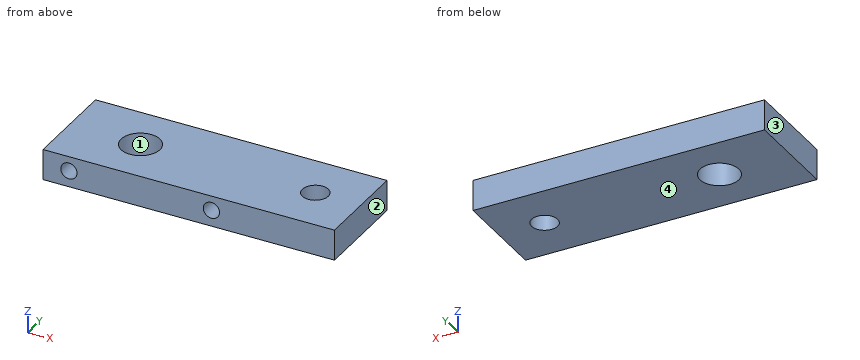
```python
from build123d import *

# Parameters (mm, degrees)
SKETCH1_W           = 90
SKETCH1_H           = 30
SKETCH1_R           = 6
SKETCH1_R_2         = 4
BOSS_EXTRUDE1_DEPTH = 9.5
SKETCH2_R           = 2.5
CUT_EXTRUDE1_DEPTH  = 15


with BuildPart() as part:
    # Sketch1 → Boss-Extrude1 (new body)
    with BuildSketch(Plane.XY):
        Rectangle(SKETCH1_W, SKETCH1_H)
        with Locations((-23, 0)):
            Circle(SKETCH1_R, mode=Mode.SUBTRACT)
        with Locations((30.98, 0)):
            Circle(SKETCH1_R_2, mode=Mode.SUBTRACT)
    extrude(amount=BOSS_EXTRUDE1_DEPTH)

    # Sketch2 → Cut-Extrude1 (cut)
    with BuildSketch(Plane.XZ.offset(15)):
        with Locations(Location((7, 5, 0), (0, 0, 270))):
            Circle(SKETCH2_R)
        with Locations(Location((-37, 5, 0), (0, 0, 270))):
            Circle(SKETCH2_R)
    extrude(amount=-CUT_EXTRUDE1_DEPTH, mode=Mode.SUBTRACT)


solid = part.part
```
The listing builds one solid part. Answer for the finished solid, in the listing's coordinates (mm). Face numbers are marked on the shaded views. Give positions to 0.01 mm unless a question says otherwise; leave off trailing zeros. Order: outer loops, then holes, each group sorted by start corner. A loop starts at its lowest first (then second) coordinate and runs counter-clockwise, first axis right, second up. Notation, with made-up numbers: (-29, 14) -> (6, 14) arc R23 ccw to (6, 50) -> close; hole circle Ø5 at (14.25, 36). An arc over 180 degrees is marked (long way). Answer as CSV lines item,"result". Start each with the question number.
Q1. A cutting plane is placed at A-A (x = 30.98). Determine the outline of the cut face in (y, z).
Q2. A cutting plane is placed at D-D (z = 1). Determine the outline of the cut face in (x, y).
Q3. A cutting plane is placed at C-C (x = 7). Determine the outline of the cut face in (y, z).
Q4. Find the intervals of material crossed by L1, parallel to X at y = -11, z = 5; L2, parallel to X at y = -0.5, z = 8.75; L3, parallel to Y at x = -23, z = 3.5, in increasing order.
Q5. Determine the mould class of the marked faces 1, 2, 3 and 4 for opening direction X: pulls with the +X half, pulls with the -X half, needs draft (parallel to the pull), parting line crosses it, or undercut.
Q6. A cutting plane is placed at B-B (z = 5). Determine the outline of the cut face in (x, y).
Q7. Given pin 1 (2.5 mm diameter, centred on x = -38, z = 5, fed in from -Y); pin 2 (5.5 mm diameter, centred on x = 7, z = 4.5, fed in from -Y), each flat-ended and moving along its own axis, determine where each tip first touches the part or whether it passes through.
Results found:
1,outline,"(-15, 0) -> (-4, 0) -> (-4, 9.5) -> (-15, 9.5) -> close; (4, 0) -> (15, 0) -> (15, 9.5) -> (4, 9.5) -> close"
2,outline,"(-45, -15) -> (45, -15) -> (45, 15) -> (-45, 15) -> close; hole circle Ø12 at (-23, 0); hole circle Ø8 at (30.98, 0)"
3,outline,"(-15, 0) -> (15, 0) -> (15, 9.5) -> (-15, 9.5) -> (-15, 7.5) -> (0, 7.5) -> (0, 2.5) -> (-15, 2.5) -> close"
4,L1,"-45 to -39.5, -34.5 to 4.5, 9.5 to 45"
4,L2,"-45 to -28.98, -17.02 to 27.01, 34.95 to 45"
4,L3,"-15 to -6, 6 to 15"
5,face 1,"undercut"
5,face 2,"pulls with the +X half"
5,face 3,"pulls with the -X half"
5,face 4,"needs draft"
6,outline,"(-45, -15) -> (-39.5, -15) -> (-39.5, 0) -> (-34.5, 0) -> (-34.5, -15) -> (4.5, -15) -> (4.5, 0) -> (9.5, 0) -> (9.5, -15) -> (45, -15) -> (45, 15) -> (-45, 15) -> close; hole circle Ø12 at (-23, 0); hole circle Ø8 at (30.98, 0)"
7,pin 1,"y = 0"
7,pin 2,"y = -15"
